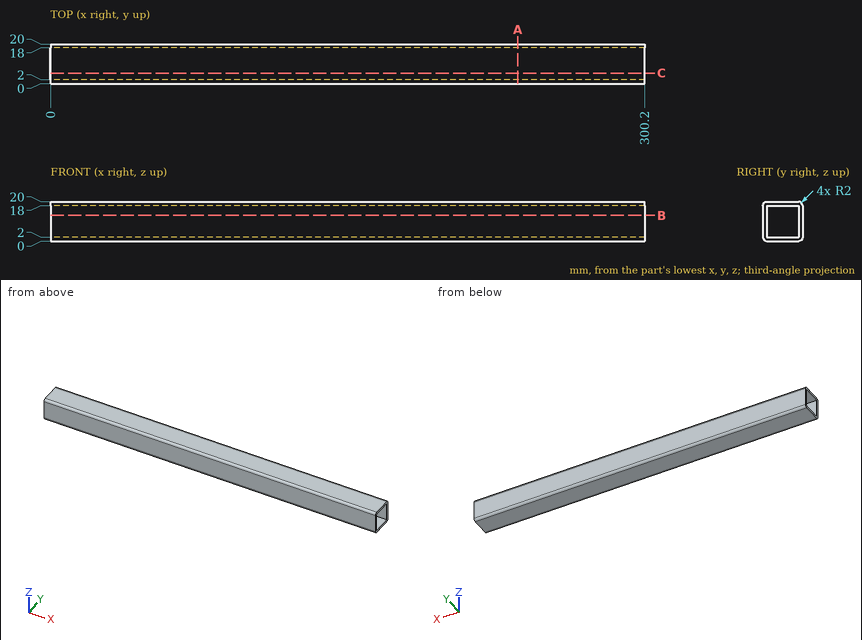
Source: three-view drawing plus pictorial views. Frame: mm from the lowest corner of the part. Coordinates: 2 decimals unless noted, no trailing zeros. Order: outer loops, then holes, each group sorted by start corner. A loop starts at its lowest first (then second) coordinate and runs counter-clockwise, first axis right, second up. Notation, with made-up numbers: M 89.25,60.25 L 132.25,60.25 A20 cw 132.25,68.25 Z; hole C 79,-18.75 d5. An arc over 180 degrees is marked long. One line per question, with ' | ' between items.
Item 1: Pin query (flat end, axial travel): pin 1 (4 mm diameter, centred on y = 16.5, z = 11.5, fed in from -X). Return the tip coordinate at first contact, or that it passes through.
Geometry results:
pin 1: stops at x = 0
Item 2: Section A-A (x = 236). Output: boundary loops of the cut face in (y, z).
Geometry results:
outline: M 0,2 A2 ccw 2,0 L 18,0 A2 ccw 20,2 L 20,18 A2 ccw 18,20 L 2,20 A2 ccw 0,18 Z; hole M 2,2 L 18,2 L 18,18 L 2,18 Z
Item 3: Ray query, line 1 along Y through (x, z) = (103.5, 14.25); line 2 along Z through (x, y) = (199, 19.25). Return the intervals inside material, ascending.
Geometry results:
line 1: y = 0 to 2, 18 to 20 | line 2: z = 0.44 to 19.56
Item 4: Section B-B (z = 13). Output: boundary loops of the cut face in (x, y).
Geometry results:
outline: M 0,0 L 300.2,0 L 300.2,2 L 0,2 Z; M 0,18 L 300.2,18 L 300.2,20 L 0,20 Z
